from build123d import *

# Parameters (mm, degrees)
CROQUIS1_W              = 85
CROQUIS1_H              = 102
CROQUIS1_R              = 4
CROQUIS1_R_2            = 2.5
CROQUIS1_R_3            = 3.15
SALIENTE_EXTRUIR1_DEPTH = 3
REDONDEO1_R             = 10


with BuildPart() as part:
    # Croquis1 → Saliente-Extruir1 (new body)
    with BuildSketch(Plane.XY):
        with Locations((11.3, 0)):
            Rectangle(CROQUIS1_W, CROQUIS1_H)
        Circle(CROQUIS1_R, mode=Mode.SUBTRACT)
        with Locations((18.25, 0)):
            Circle(CROQUIS1_R_2, mode=Mode.SUBTRACT)
        with Locations(Location((-18.25, 0, 0), (0, 0, 180))):
            Circle(CROQUIS1_R_2, mode=Mode.SUBTRACT)
        with Locations((-9.5, 38.5)):
            Circle(CROQUIS1_R_3, mode=Mode.SUBTRACT)
        with Locations(Location((-9.5, -38.5, 0), (0, 0, 180))):
            Circle(CROQUIS1_R_3, mode=Mode.SUBTRACT)
        with Locations((41.3, 38.5)):
            Circle(CROQUIS1_R_3, mode=Mode.SUBTRACT)
        with Locations(Location((41.3, -38.5, 0), (0, 0, 180))):
            Circle(CROQUIS1_R_3, mode=Mode.SUBTRACT)
    extrude(amount=SALIENTE_EXTRUIR1_DEPTH)

    # Redondeo1
    redondeo1_edges = [part.edges().sort_by_distance(p)[0] for p in [
        (-31.2, 51, 1.5),
        (53.8, 51, 1.5),
        (53.8, -51, 1.5),
        (-31.2, -51, 1.5),
    ]]
    fillet(redondeo1_edges, radius=REDONDEO1_R)


solid = part.part
Input: part model. Units: mm. Frame: model coordinates. Coordinates: 2 decimals unless noted, no trailing zeros. Loops run counter-clockwise (first coordinate to the right, second up) from the corner with the lowest first, then second, coordinate; pieces in that order, holes last.
Q1. Cut plane D-D (z = 1). Output: boundary loops of the cut face in (x, y), then the cut area to 3 significant figures.
Q2. Material intervals for line 1 (Y direction, x = -9.5, z = 1.6); line 2 (X direction, y = -38.5, z = 0.7); line 3 (Y direction, x = 18.25, z = 1.15), sorted ascending.
Q3. Contact query for flat-ended pins moving along their axis: pin 1 (1 mm diameter, centred on x = 27.5, y = -9.5, fed in from -Z); pin 2 (4 mm diameter, centred on x = -18.25, y = 0, fed in from +Z). Output: stop coordinate, or through.
Q4. Cut plane A-A (x = 0). Output: boundary loops of the cut face in (y, z), then the cut area to 3 significant figures.
Q5. Draft query along Y for faces 1 (the face through (11, -51, 1)), 2 (the face through (15.752, 0.11, 1.479)), 3 (the face through (53.8, -1, 1)), 4 (the face through (41.983, -35.425, 1.479)). Return one class per face: +Y half, -Y half, draft (parallel to the pull), parting line (faces both ways), or undercut.
Q6. Cut plane C-C (x = 41.3). Output: boundary loops of the cut face in (y, z), then the cut area to 3 significant figures.
Q7. Cut plane B-B (y = 0). Output: boundary loops of the cut face in (x, z).
Working result:
1. outline: (-31.2, -41) arc R10 ccw to (-21.2, -51) - (43.8, -51) arc R10 ccw to (53.8, -41) - (53.8, 41) arc R10 ccw to (43.8, 51) - (-21.2, 51) arc R10 ccw to (-31.2, 41) - close; hole circle Ø5 at (-18.25, 0); hole circle Ø6.3 at (-9.5, -38.5); hole circle Ø6.3 at (-9.5, 38.5); hole circle Ø8 at (0, 0); hole circle Ø5 at (18.25, 0); hole circle Ø6.3 at (41.3, -38.5); hole circle Ø6.3 at (41.3, 38.5)
1. area: 8,370 mm2
2. line 1: y = -51 to -41.65, -35.35 to 35.35, 41.65 to 51
2. line 2: x = -31.2 to -12.65, -6.35 to 38.15, 44.45 to 53.8
2. line 3: y = -51 to -2.5, 2.5 to 51
3. pin 1: stops at z = 0
3. pin 2: passes through
4. outline: (-51, 0) - (-4, 0) - (-4, 3) - (-51, 3) - close; (4, 0) - (51, 0) - (51, 3) - (4, 3) - close
4. area: 282 mm2
5. face 1: -Y half
5. face 2: undercut
5. face 3: draft
5. face 4: undercut
6. outline: (-51, 0) - (-41.65, 0) - (-41.65, 3) - (-51, 3) - close; (-35.35, 0) - (35.35, 0) - (35.35, 3) - (-35.35, 3) - close; (41.65, 0) - (51, 0) - (51, 3) - (41.65, 3) - close
6. area: 268 mm2
7. outline: (-31.2, 0) - (-20.75, 0) - (-20.75, 3) - (-31.2, 3) - close; (-15.75, 0) - (-4, 0) - (-4, 3) - (-15.75, 3) - close; (4, 0) - (15.75, 0) - (15.75, 3) - (4, 3) - close; (20.75, 0) - (53.8, 0) - (53.8, 3) - (20.75, 3) - close
